Source: CAD feature listing. Evaluate the final solid. Frame: model axes, mm. Face numbers are marked on the shaded views. A direction names the side the tool comes from. Give positions to 0.01 mm unless a question says otherwise; leave off trailing zeros. Loops run counter-clockwise (first coordinate to the right, second up) from the corner with the lowest first, then second, coordinate; pieces in that order, holes last.
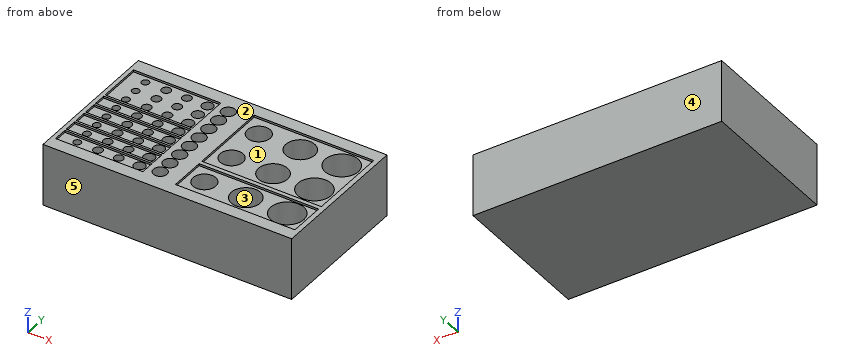
```python
from build123d import *

# Parameters (mm, degrees)
SKETCH_W               = 120
SKETCH_H               = 70
PAD_DEPTH              = 30
SKETCH001_R            = 2.2
SKETCH001_R_2          = 3.3
SKETCH001_R_3          = 2.7
SKETCH001_R_4          = 1.8
POCKET_DEPTH           = 12
LINEARPATTERN_COUNT    = 8
LINEARPATTERN_PITCH    = 7.142857
SKETCH002_R            = 5.5
SKETCH002_R_2          = 7
SKETCH002_R_3          = 8
POCKET001_DEPTH        = 25
LINEARPATTERN001_COUNT = 3
LINEARPATTERN001_PITCH = 20
SKETCH003_W            = 42.132603
SKETCH003_H            = 20.915248
SKETCH003_H_2          = 6.049934
SKETCH003_H_3          = 6.286621
SKETCH003_H_4          = 6.053579
SKETCH003_H_5          = 6.157676
SKETCH003_H_6          = 6.848442
SKETCH003_W_2          = 57.669466
SKETCH003_H_7          = 38.496372
SKETCH003_H_8          = 17.364103
POCKET002_DEPTH        = 1


with BuildPart() as part:
    # Sketch → Pad (new body)
    with BuildSketch(Plane.XY):
        Rectangle(SKETCH_W, SKETCH_H)
    extrude(amount=PAD_DEPTH)

    # Sketch001 → Pocket (cut)
    with BuildSketch(Plane.XY.offset(30)):
        with Locations((-40, 25)):
            Circle(SKETCH001_R)
        with Locations((-10, 25)):
            Circle(SKETCH001_R_2)
        with Locations((-30, 25)):
            Circle(SKETCH001_R)
        with Locations((-20, 25)):
            Circle(SKETCH001_R_3)
        with Locations((-50, 25)):
            Circle(SKETCH001_R_4)
    pocket = extrude(amount=-POCKET_DEPTH, mode=Mode.SUBTRACT)

    # LinearPattern: Pocket ×8
    with Locations(*[(0, -i * LINEARPATTERN_PITCH, 0) for i in range(1, LINEARPATTERN_COUNT)]):
        add(pocket, mode=Mode.SUBTRACT)

    # Sketch002 → Pocket001 (cut)
    with BuildSketch(Plane.XY.offset(30)):
        with Locations((8, -20)):
            Circle(SKETCH002_R)
        with Locations((28, -20)):
            Circle(SKETCH002_R_2)
        with Locations((48, -20)):
            Circle(SKETCH002_R_3)
    pocket001 = extrude(amount=-POCKET001_DEPTH, mode=Mode.SUBTRACT)

    # LinearPattern001: Pocket001 ×3
    with Locations(*[(0, i * LINEARPATTERN001_PITCH, 0) for i in range(1, LINEARPATTERN001_COUNT)]):
        add(pocket001, mode=Mode.SUBTRACT)

    # Sketch003 → Pocket002 (cut)
    with BuildSketch(Plane.XY.offset(30)):
        with Locations((-36.933698, 18.03323)):
            Rectangle(SKETCH003_W, SKETCH003_H)
        with Locations((-36.933698, 3.550639)):
            Rectangle(SKETCH003_W, SKETCH003_H_2)
        with Locations((-36.933698, -3.617638)):
            Rectangle(SKETCH003_W, SKETCH003_H_3)
        with Locations((-36.933698, -10.787738)):
            Rectangle(SKETCH003_W, SKETCH003_H_4)
        with Locations((-36.933698, -17.893366)):
            Rectangle(SKETCH003_W, SKETCH003_H_5)
        with Locations((-36.933698, -25.396425)):
            Rectangle(SKETCH003_W, SKETCH003_H_6)
        with Locations((28.834733, 9.552328)):
            Rectangle(SKETCH003_W_2, SKETCH003_H_7)
        with Locations((28.834733, -20.377909)):
            Rectangle(SKETCH003_W_2, SKETCH003_H_8)
    extrude(amount=-POCKET002_DEPTH, mode=Mode.SUBTRACT)


solid = part.part
```
(1) Reachability of the marked faces 1 and 2 from +Z, -Z, +X, -X, +Y, -Y: full face, straight path, thin tool, end or side. Return the list, or none.
A:
face 1: +Z
face 2: +Z, +X, -X, +Y, -Y
(2) First-contact query: pin 1 (7 mm diameter, centred on x = -20, y = 17.86, fed in from +Z); pin 2 (5 mm diameter, centred on x = 48, y = 4.5, fed in from +Z); pin 3 (1.6 mm diameter, centred on x = -19.5, y = -2.5, fed in from +Z); pin 4 (1 mm diameter, centred on x = 3, y = -3, fed in from -Z). Flat tips, straight axial feed; report the tip coordinate or a pass-through.
A:
pin 1: stops at z = 29
pin 2: stops at z = 5
pin 3: stops at z = 18
pin 4: stops at z = 0
(3) Section B-B, the plane x = 47.5. Return the cut outline in (y, z), then the cut area to 3 significant figures.
A:
outline: (-35, 0) - (35, 0) - (35, 30) - (28.8, 30) - (28.8, 29) - (27.98, 29) - (27.98, 5) - (12.02, 5) - (12.02, 29) - (7.98, 29) - (7.98, 5) - (-7.98, 5) - (-7.98, 29) - (-9.7, 29) - (-9.7, 30) - (-11.7, 30) - (-11.7, 29) - (-12.02, 29) - (-12.02, 5) - (-27.98, 5) - (-27.98, 29) - (-29.06, 29) - (-29.06, 30) - (-35, 30) - close
area: 894 mm2
(4) Section A-A, the plane z = 8. Count the separate pieces of the cut face and the enclosed holes in it, then the cut area to 3 significant figures.
A:
separate pieces: 1
enclosed holes: 9
area: 7,050 mm2
(5) Mould query, pull axis Y, two halves, no side actions, for the marked faces 3, 4 and 5. Classes: pulls with the +Y half, pulls with the -Y half, needs draft (parallel to the pull), parting line crosses it, or undercut.
A:
face 3: undercut
face 4: pulls with the +Y half
face 5: pulls with the -Y half
(6) Ray query, line 1 along Y through (x, z) = (28, 12.75); line 2 along Y through (x, z) = (8.5, 8); line 3 along X through (y, z) = (21.5, 15.75). Return the intervals inside material, ascending.
A:
line 1: y = -35 to -27, -13 to -7, 7 to 13, 27 to 35
line 2: y = -35 to -25.48, -14.52 to -5.48, 5.48 to 14.52, 25.48 to 35
line 3: x = -60 to 2.71, 13.29 to 21.16, 34.84 to 40.14, 55.86 to 60
